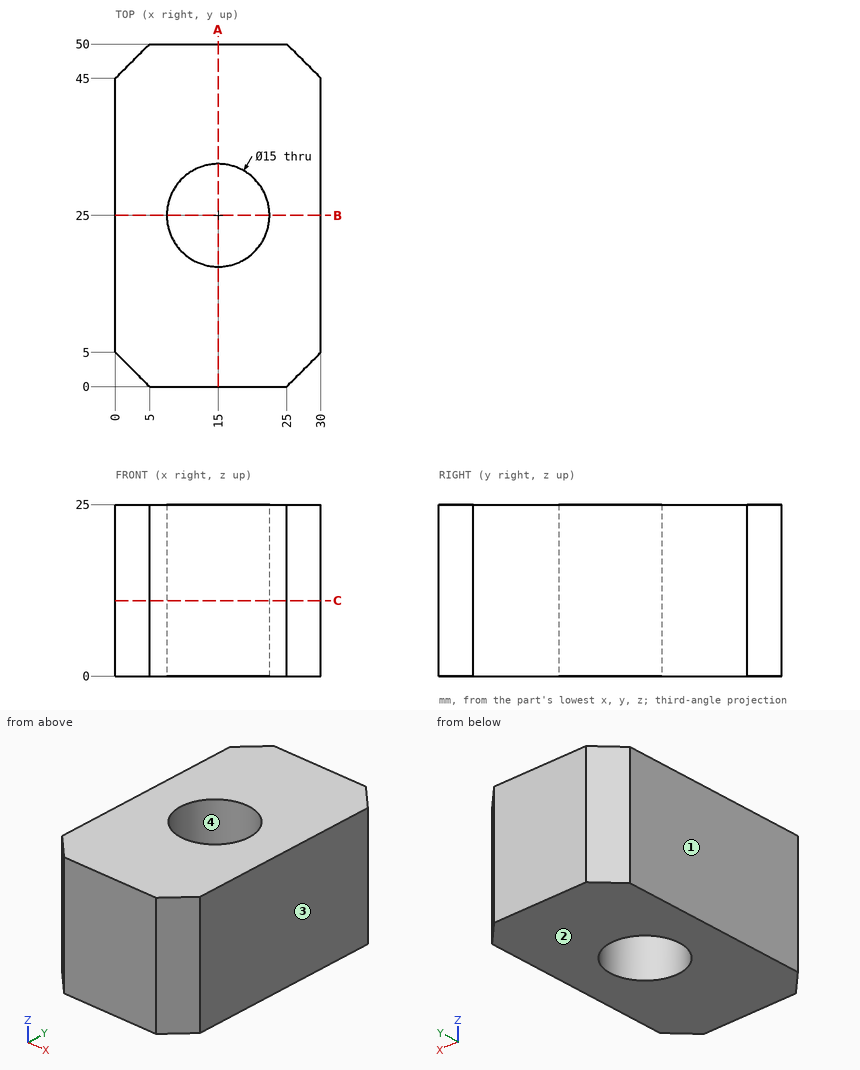
Here's the drawing with two shaded views (mm, measured from the low corner). I have some questions. Give positions to 0.01 mm unless a question says otherwise; leave off trailing zeros. Write each loop counter-clockwise with the first axis right and the second up, starting at its lowest first coordinate (ties: lowest second). Pieces come first, ordered by that corner, then holes. Notation, with made-up numbers: (43.25, 81.5) - (83.25, 81.5) arc R25 ccw to (83.25, 111.5) - close; hole circle Ø8 at (-6, 74.5). An arc over 180 degrees is marked (long way). One line per item, written item: value. Start each with the question number.
Item 1: Please list where these lines run through material, in increasing order: line 1 (Y direction, x = 15, z = 9.75); line 2 (Y direction, x = 8.25, z = 20.75); line 3 (X direction, y = 31, z = 11.75). Write a range as from..to.
Item 2: Imagine slicing it at B-B, the plane y = 25. List the corners of the cut face in (x, z) for me, and give its area (3 significant figures).
Item 3: If we mould it in two halves opening along X, with no side actions, what happens to the marked faces 1, 2, 3 and 4? For each: +X half, -X half, draft (parallel to the pull), parting line (faces both ways), or undercut.
Item 4: Imagine slicing it at C-C, the plane z = 11. List the corners of the cut face in (x, y) for me, and give its area (3 significant figures).
Item 5: I'm going to push a flat-ended pin straight in: pin 1 (1 mm diameter, centred on x = 3, z = 9.5, fed in from +Y). Where does the tip first touch, or does it pass through?
Item 6: Imagine slicing it at A-A, the plane x = 15. List the corners of the cut face in (y, z) for me.
Geometry says:
1. line 1: 0..17.5, 32.5..50
1. line 2: 0..21.73, 28.27..50
1. line 3: 0..10.5, 19.5..30
2. outline: (0, 0) - (7.5, 0) - (7.5, 25) - (0, 25) - close; (22.5, 0) - (30, 0) - (30, 25) - (22.5, 25) - close
2. area: 375 mm^2
3. face 1: -X half
3. face 2: draft
3. face 3: +X half
3. face 4: undercut
4. outline: (0, 5) - (5, 0) - (25, 0) - (30, 5) - (30, 45) - (25, 50) - (5, 50) - (0, 45) - close; hole circle Ø15 at (15, 25)
4. area: 1,270 mm^2
5. pin 1: y = 48.5
6. outline: (0, 0) - (17.5, 0) - (17.5, 25) - (0, 25) - close; (32.5, 0) - (50, 0) - (50, 25) - (32.5, 25) - close
